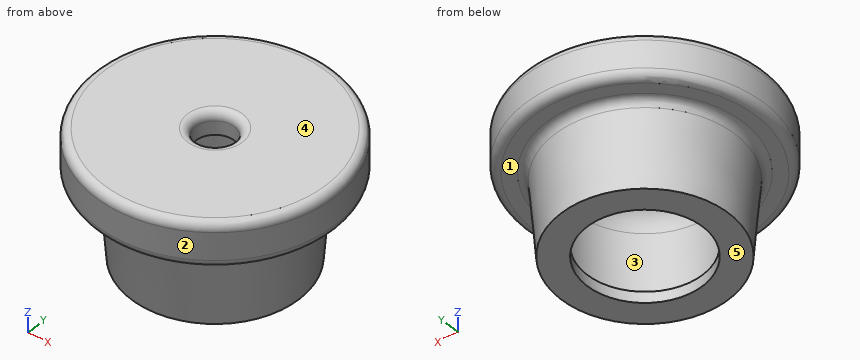
```python
from build123d import *

# Parameters (mm, degrees)
F2_R = 1.5
F3_R = 5


with BuildPart() as f1:
    # F0 (on Front) → F1 (revolve)
    with BuildSketch(Plane.XZ):
        Polygon((21.7, 11.509762), (3.5, 11.509762), (3.5, 7.509762), (12.506023, 7.509762), (12.506023, -9.490238), (10.506023, -9.490238), (10.506023, -11.490238), (15.25, -11.490238), (16.5, 3.509762), (21.7, 3.509762), align=None)
    revolve(axis=Axis((0, 0, -6.313648), (0, 0, -1)))

    # F2
    f2_edges = [f1.edges().sort_by_distance(p)[0] for p in [
        (-3.5, 0, 11.509762),
        (-21.7, 0, 11.509762),
        (-21.7, 0, 3.509762),
        (-16.5, 0, 3.509762),
    ]]
    fillet(f2_edges, radius=F2_R)

    # F3
    f3_edges = [f1.edges().sort_by_distance(p)[0] for p in [
        (-12.506023, 0, 7.509762),
    ]]
    fillet(f3_edges, radius=F3_R)


solid = f1.part
```
Verification items for the finished model (mm, model axes). Face numbers are marked on the shaded views. A direction names the side the tool comes from. Round coordinates to 2 decimals unless told otherwise and drop trailing zeros. Order: outer loops, then holes, each group sorted by start corner. A loop starts at its lowest first (then second) coordinate and runs counter-clockwise, first axis right, second up.
1) Cross-section at D-D, the plane z = 6. Record the cut outline in (x, y).
Geometry says:
outline: circle Ø43.4 at (0, 0); hole circle Ø22.17 at (0, 0)
2) Cross-section at C-C, the plane z = -1.5. Record the cut outline in (x, y).
Geometry says:
outline: circle Ø32.17 at (0, 0); hole circle Ø25.01 at (0, 0)
3) Tool access check on the marked faces 1 and 2. Record the directions out of +Z, -Z, +X, -X, +Y, -Y that give a thin tool (end or side, any length) a straight path to the whole face; none if there is none.
Geometry says:
face 1: -Z
face 2: +Z, -Z
4) Material ranges on line 1 (Y direction, x = 0, z = 8.7); line 2 (Y direction, x = -8.5, z = 0); line 3 (X direction, y = -0.5, z = -8.5), recorded low to high.
Geometry says:
line 1: y = -21.7 to -3.5, 3.5 to 21.7
line 2: y = -13.8 to -9.17, 9.17 to 13.8
line 3: x = -15.49 to -12.5, 12.5 to 15.49
5) Depth check by flat-ended pin: pin 1 (3 mm diameter, centred on y = -3.5, z = -4.5, fed in from +X); pin 2 (3 mm diameter, centred on y = 6, z = -4, fed in from -X); pin 3 (1 mm diameter, centred on x = 3, z = -1, fed in from -Y). Enter the tip coordinate at first touch or a pass-through.
Geometry says:
pin 1: stops at x = 15.74
pin 2: stops at x = -15.24
pin 3: stops at y = -15.94
6) Draft check along Z on the marked faces 3, 4 and 5. Enter one of: +Z half, -Z half, draft (parallel to the pull), parting line (faces both ways), or undercut.
Geometry says:
face 3: undercut
face 4: +Z half
face 5: -Z half
